from build123d import *

# Parameters (mm, degrees)
F1_DEPTH = 9.398
F2_DEPTH = 5.08
F3_R     = 1.524
F4_DEPTH = 6.6633576407
F5_R     = 1.27


with BuildPart() as f1:
    # F0 (on Top) → F1 (new body)
    with BuildSketch(Plane.XY):
        with BuildLine():
            ThreePointArc((-10.8032145216, -5.08), (-11.6508501612, -2.6026014909), (-11.938, 0))
            Line((-11.938, 0), (-19.558, 0))
            Line((-19.558, 0), (-19.558, -5.08))
            Line((-19.558, -5.08), (-10.8032145216, -5.08))
        make_face()
        with BuildLine():
            ThreePointArc((8.128, 0), (0, -8.128), (-8.128, 0))
            Line((-8.128, 0), (-11.938, 0))
            ThreePointArc((-11.938, 0), (-11.6508501612, -2.6026014909), (-10.8032145216, -5.08))
            ThreePointArc((-10.8032145216, -5.08), (0, -11.938), (10.8032145216, -5.08))
            ThreePointArc((10.8032145216, -5.08), (11.6508501612, -2.6026014909), (11.938, 0))
            Line((11.938, 0), (8.128, 0))
        make_face()
        with BuildLine():
            Line((19.558, 0), (11.938, 0))
            ThreePointArc((11.938, 0), (11.6508501612, -2.6026014909), (10.8032145216, -5.08))
            Line((10.8032145216, -5.08), (19.558, -5.08))
            Line((19.558, -5.08), (19.558, 0))
        make_face()
    extrude(amount=F1_DEPTH)

    # F0 (on Top) → F2 (join)
    with BuildSketch(Plane.XY):
        with BuildLine():
            ThreePointArc((5.842, 0), (0, -5.842), (-5.842, 0))
            Line((-5.842, 0), (-8.128, 0))
            ThreePointArc((-8.128, 0), (0, -8.128), (8.128, 0))
            Line((8.128, 0), (5.842, 0))
        make_face()
    extrude(amount=F2_DEPTH)

    # F3 (on face) → F4 (cut, through all)
    with BuildSketch(Plane(origin=(0, 0, 0), x_dir=(-1, 0, 0), z_dir=(0, 1, 0))):
        with Locations((-11.43, 5.715)):
            Circle(F3_R)
        with Locations((11.43, 5.715)):
            Circle(F3_R)
    extrude(amount=-F4_DEPTH, mode=Mode.SUBTRACT)

    # F5
    f5_edges = [f1.edges().sort_by_distance(p)[0] for p in [
        (5.842, 0, 2.54),
        (-5.842, 0, 2.54),
        (8.128, 0, 7.239),
        (-8.128, 0, 7.239),
        (19.558, 0, 4.699),
        (19.558, -5.08, 4.699),
        (-19.558, 0, 4.699),
        (-19.558, -5.08, 4.699),
    ]]
    fillet(f5_edges, radius=F5_R)


solid = f1.part
Part model, mm, in its own coordinate system. A direction names the side the tool comes from. Coordinates: 2 decimals unless noted, no trailing zeros. Loops run counter-clockwise (first coordinate to the right, second up) from the corner with the lowest first, then second, coordinate; pieces in that order, holes last. Notation, with made-up numbers: M 86.25,49 L 129.25,49 A31 cw 129.25,83 Z; hole C 88.5,-3 d9. An arc over 180 degrees is marked long. Use a Markdown table: item, result. Add a question column.
Q1. Cut at A-A (x = 11.43). Write the cut outline in (y, z), and give its area (3 significant figures).
Q2. Probe L1, parallel to Z at x = 11.43, y = -3.25; L2, parallel to X at y = -1, z = 6.75; L3, parallel to Y at x = 13.5, z = 6. List the from-to ranges inside material, lowest first.
Q3. Cut at C-C (z = 8.5). Write the cut outline in (x, y), and give its area (3 significant figures).
Q4. Which spindle directions (+Z, -Z, +X, -X, +Y, -Y) get a long thin tool onto all of the face, cutting with end or side? Do faces 1 (the cylindrical face through (-8.49, -0.3, 7.27)), 2 (the cylindrical face through (-6.174, -0.303, 2.576)), 3 (the cylindrical face through (9.976, -2.544, 6.173)), 4 (the flat face through (-15, -5.08, 5)), 5 (the flat face through (0, -9, 9.398)). Say none if no direction does.
Q5. Pin check, flat tips, straight feed: P1, Ø2, axis at x = -15, z = 5, coming from the -Y side; P2, Ø6, axis at x = -5.5, y = -6, coming from the -Z side. Stop position of each tip, or through.
Q6. Cut at B-B (y = -5.5). Write the cut outline in (x, z) (1 decimal).
Q7. Mould opens along X. For faces 6 (the cylindrical face through (0.11, -5.84, 2.5)), 7 (the cylindrical face through (19.196, -4.698, 4.765)), 8 (the flat face through (14, -5.08, 5)) say: +X half, -X half, draft (parallel to the pull), parting line (faces both ways), or undercut.
Q8. Cut at D-D (y = -7.25). Write the cut outline in (x, z), and give its area (3 significant figures).
Worked out:
| question | item | result |
|---|---|---|
| 1 | outline | M -5.08,0 L 0,0 L 0,4.19 L -5.08,4.19 Z; M -5.08,7.24 L 0,7.24 L 0,9.4 L -5.08,9.4 Z |
| 1 | area | 32.3 mm2 |
| 2 | L1 | z = 0 to 4.19, 7.24 to 9.4 |
| 2 | L2 | x = -19.53 to -12.55, -10.31 to -8.07, 8.07 to 10.31, 12.55 to 19.53 |
| 2 | L3 | y = -5.08 to 0 |
| 3 | outline | M -19.56,-3.81 A1.27 ccw -18.29,-5.08 L -10.8,-5.08 A11.94 ccw 10.8,-5.08 L 18.29,-5.08 A1.27 ccw 19.56,-3.81 L 19.56,-1.27 A1.27 ccw 18.29,0 L 9.31,0 A1.27 ccw 8.05,-1.1 A8.13 cw -8.05,-1.1 A1.27 ccw -9.31,0 L -18.29,0 A1.27 ccw -19.56,-1.27 Z |
| 3 | area | 199 mm2 |
| 4 | face 1 | +Z, +Y |
| 4 | face 2 | +Z, -Z, +Y |
| 4 | face 3 | +Y, -Y |
| 4 | face 4 | +Z, -Z, -X, -Y |
| 4 | face 5 | +Z, +X, -X, +Y, -Y |
| 5 | P1 | stops at y = -5.08 |
| 5 | P2 | stops at z = 0 |
| 6 | outline | M -10.6,0 L -2,0 L -2,5.1 L -6,5.1 L -6,9.4 L -10.6,9.4 L -10.6,7 A1.5 cw -10.6,4.4 Z; M 2,0 L 10.6,0 L 10.6,4.4 A1.5 cw 10.6,7 L 10.6,9.4 L 6,9.4 L 6,5.1 L 2,5.1 Z |
| 7 | face 6 | undercut |
| 7 | face 7 | +X half |
| 7 | face 8 | draft |
| 8 | outline | M -9.48,0 L 9.48,0 L 9.48,9.4 L 3.67,9.4 L 3.67,5.08 L -3.67,5.08 L -3.67,9.4 L -9.48,9.4 Z |
| 8 | area | 147 mm2 |
